from build123d import *

# Parameters (mm, degrees)
F1_ANGLE = 180
F2_W     = 16.51
F2_H     = 2.667
F3_DEPTH = 25.4
F2_W_2   = 4.643438
F4_DEPTH = 19.05


with BuildPart() as f1:
    # F0 (on Front) → F1 (revolve)
    with BuildSketch(Plane.XZ):
        Polygon((16.073437, -3.344848), (16.073438, -98.594848), (22.423438, -98.594848), (22.423438, 9.355152), (0, 9.355152), (0, -16.044848), (12.501562, -16.044848), (12.501562, -3.344848), align=None)
    revolve(axis=Axis((0, 0, -3.344848), (0, 0, -1)), revolution_arc=F1_ANGLE)

    # F2 (on face) → F3 (cut, through all)
    with BuildSketch(Plane.XY.offset(9.355152)):
        with Locations((0, -1.3335)):
            Rectangle(F2_W, F2_H)
    extrude(amount=-F3_DEPTH, mode=Mode.SUBTRACT)

    # F2 (on face) → F4 (cut)
    with BuildSketch(Plane.XY.offset(9.355152)):
        with Locations((10.576719, -1.3335)):
            Rectangle(F2_W_2, F2_H)
        with Locations((-10.576719, -1.3335)):
            Rectangle(F2_W_2, F2_H)
    extrude(amount=-F4_DEPTH, mode=Mode.SUBTRACT)


solid = f1.part
The listing builds one solid part. Answer for the finished solid, in the listing's coordinates (mm). A direction names the side the tool comes from. Coordinates: 2 decimals unless noted, no trailing zeros. Loops run counter-clockwise (first coordinate to the right, second up) from the corner with the lowest first, then second, coordinate; pieces in that order, holes last. Notation, with made-up numbers: (-7, -28) -> (3, -28) arc R5 cw to (3, -21) -> close; hole circle Ø7 at (32.5, 57.25). An arc over 180 degrees is marked (long way). Write item = value, one per line. Start each with the question number.
1) Given pin 1 Ø10 at (y, z) = (-7, -69.5) entering from +X; pin 2 Ø1.3 at (y, z) = (-1.5, -12) entering from -X; pin 3 Ø10 at (x, y) = (3.5, -8) entering from -Z; pin 4 Ø1 at (x, y) = (16.5, -17) entering from -Z, each flat-ended and moving along its own axis, determine where each tip first touches the part or whether it passes through.
2) A cutting plane is placed at A-A (z = -13). Give the vertices of the cut face in (x, y) (3 decimals), then the cut area to 3 significant figures.
3) A cutting plane is placed at D-D (z = -24). Give the vertices of the cut face in (x, y).
4) A tool of negligible diameter and unlimited length cuts with its end or side. For faces 1 (the face through (-10, -1, -9.695)), 2 (the face through (-1, -13, -3.345)), 3 (the face through (8.255, -1, -13)), from which of +Z, -Z, +X, -X, +Y, -Y can it reach the whole face along a straight path? Write none if from no direction.
5) A cutting plane is placed at B-B (x = 0). Give the vertices of the cut face in (y, z), then the cut area to 3 significant figures.
6) A cutting plane is placed at C-C (y = -8.75). Give the vertices of the cut face in (x, z), then the cut area to 3 significant figures.
7) The mould has two halves that part along Y. Classify faces 4 (the face through (0.27, -12.5, -9.61)), 5 (the face through (0, -11, 9.355)), 6 (the face through (0.49, -22.42, -43.86)): released by +Y, released by -Y, zero draft, split by the parting line, or undercut.
8) Straight lines are drawn through the part: line 1 (X direction, y = -6, z = -13.5); line 2 (X direction, y = -1.25, z = -83); line 3 (Z direction, x = 2.5, y = -9). For each, find the intervals that lie inside material, in ascending order. Write a range as from..to.
Responses:
q1.pin_1 = 22.33
q1.pin_2 = -22.41
q1.pin_3 = -16.04
q1.pin_4 = through
q2.outline = (-22.423, 0) arc R22.423 ccw to (22.423, 0) -> (16.073, 0) arc R16.073 cw to (-16.073, 0) -> close; (-12.502, 0) arc R12.502 ccw to (12.502, 0) -> (8.255, 0) -> (8.255, -2.667) -> (-8.255, -2.667) -> (-8.255, 0) -> close
q2.area = 585 mm²
q3.outline = (-22.42, 0) arc R22.42 ccw to (22.42, 0) -> (16.07, 0) arc R16.07 cw to (-16.07, 0) -> close
q4.face_1 = +Z, +Y
q4.face_2 = -Z
q4.face_3 = +Z, -Z, +Y
q5.outline = (-22.42, -98.59) -> (-16.07, -98.59) -> (-16.07, -3.34) -> (-12.5, -3.34) -> (-12.5, -16.04) -> (-2.67, -16.04) -> (-2.67, 9.36) -> (-22.42, 9.36) -> close
q5.area = 981 mm²
q6.outline = (-20.65, -98.59) -> (-13.48, -98.59) -> (-13.48, -3.34) -> (-8.93, -3.34) -> (-8.93, -16.04) -> (8.93, -16.04) -> (8.93, -3.34) -> (13.48, -3.34) -> (13.48, -98.59) -> (20.65, -98.59) -> (20.65, 9.36) -> (-20.65, 9.36) -> close
q6.area = 2,120 mm²
q7.face_4 = undercut
q7.face_5 = zero draft
q7.face_6 = released by -Y
q8.line_1 = -21.61..-14.91, -10.97..10.97, 14.91..21.61
q8.line_2 = -22.39..-16.02, 16.02..22.39
q8.line_3 = -16.04..9.36
